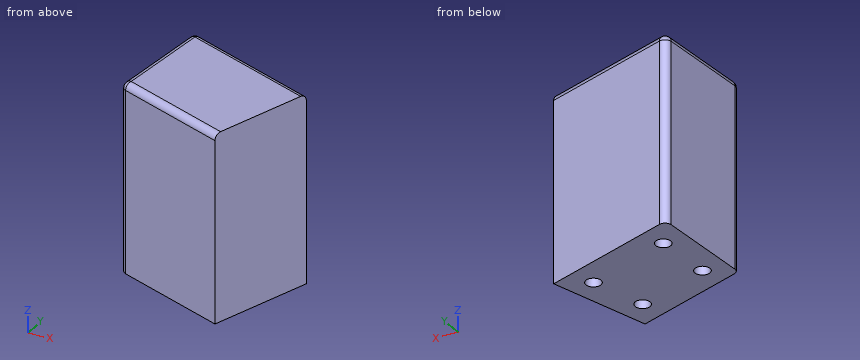
from build123d import *

# Parameters (mm, degrees)
BOSS_EXTRUDE1_DEPTH       = 74.025
FILLET1_R                 = 2.54
HOLE1_AT_2_COUNT          = 2
HOLE1_AT_2_PITCH          = 35.650433853
HOLE1_AT_3_COUNT          = 2
HOLE1_AT_3_PITCH          = 37.7542539
HOLE1_AT_4_COUNT          = 2
HOLE1_AT_4_PITCH          = 22.225
F_8_CLEARANCE_HOLE1_D     = 4.9149
F_8_CLEARANCE_HOLE1_DEPTH = 12.7
F_8_CLEARANCE_HOLE1_TIP   = 1.476584928


with BuildPart() as part:
    # Sketch1 → Boss-Extrude1 (new body)
    with BuildSketch(Plane.XY):
        Polygon((277.604402796, 374.816405204), (281.415155825, 417.005352091), (335.71810759, 399.192100573), (322.852981494, 359.973302076), align=None)
    extrude(amount=BOSS_EXTRUDE1_DEPTH)

    # Fillet1
    fillet1_edges = [part.edges().sort_by_distance(p)[0] for p in [
        (281.415155825, 417.005352091, 37.0125),
        (279.509779311, 395.910878647, 74.025),
        (300.228692145, 367.39485364, 74.025),
        (308.566631708, 408.098726332, 74.025),
        (277.604402796, 374.816405204, 37.0125),
    ]]
    fillet(fillet1_edges, radius=FILLET1_R)

    # Sketch3 → Hole1 (revolve, cut)
    with BuildSketch(Plane(origin=(323.698740376, 393.110483865, 0), x_dir=(0, 1, 0), z_dir=(1, 0, 0))):
        Polygon((0, 0), (0, 4.699), (2.8702, 4.699), (2.9972, 0), align=None)
    hole1 = revolve(axis=Axis((323.698740376, 393.110483865, 110), (0, 0, -1)), mode=Mode.SUBTRACT)

    # Hole1 at 2: Hole1 ×2
    with Locations(*[Vector(-0.950182883, 0.31169294, 0) * (i * HOLE1_AT_2_PITCH) for i in range(1, HOLE1_AT_2_COUNT)]):
        add(hole1, mode=Mode.SUBTRACT)

    # Hole1 at 3: Hole1 ×2
    with Locations(*[Vector(-0.951584848, -0.307386202, 0) * (i * HOLE1_AT_3_PITCH) for i in range(1, HOLE1_AT_3_COUNT)]):
        add(hole1, mode=Mode.SUBTRACT)

    # Hole1 at 4: Hole1 ×2
    with Locations(*[Vector(-0.31169294, -0.950182883, 0) * (i * HOLE1_AT_4_PITCH) for i in range(1, HOLE1_AT_4_COUNT)]):
        add(hole1, mode=Mode.SUBTRACT)

    # #8 Clearance Hole1
    with Locations(Plane(origin=(0, 0, 0), x_dir=(-1, 0, 0), z_dir=(0, 0, -1))):
        with Locations((-323.698740376, 393.110483865), (-289.824308357, 404.222472403), (-287.772364418, 381.505347156), (-316.771364786, 371.99266929)):
            Hole(F_8_CLEARANCE_HOLE1_D / 2, depth=F_8_CLEARANCE_HOLE1_DEPTH)
            with Locations((0, 0, -(F_8_CLEARANCE_HOLE1_DEPTH + F_8_CLEARANCE_HOLE1_TIP / 2))):  # 118° drill point
                Cone(0, F_8_CLEARANCE_HOLE1_D / 2, F_8_CLEARANCE_HOLE1_TIP, mode=Mode.SUBTRACT)


solid = part.part
Model file for the job. Use its own axes, mm. Round coordinates to 2 decimals unless told otherwise and drop trailing zeros. Order: outer loops, then holes, each group sorted by start corner. A loop starts at its lowest first (then second) coordinate and runs counter-clockwise, first axis right, second up.
(1) Band-saw the part on A-A (z = 69). List the corners of the cut face in (x, y).
(2) Drill centre lines: line 1 (Y direction, x = 316.5, z = 5); line 2 (X direction, y = 391.5, z = 7); line 3 (Z direction, x = 289, y = 384) (3 decimals). Where is each one in solid material? Low to high.
(3) Pin check, flat tips, straight feed: pin 1 (1.7 mm diameter, centred on x = 290, y = 404, fed in from -Z); pin 2 (3 mm diameter, centred on x = 289.82, y = 404.22, fed in from -Z); pin 3 (2 mm diameter, centred on y = 391, z = 53, fed in from +X). Stop position of each tip, or through.
Verdict:
1. outline: (277.79, 376.83) arc R2.54 ccw to (279.52, 374.19) - (322.85, 359.97) - (335.72, 399.19) - (284.45, 416.01) arc R2.54 ccw to (281.13, 413.83) - close
2. line 1: y = 362.06 to 369.55, 374.44 to 405.5
2. line 2: x = 279.11 to 321.84, 325.55 to 333.19
2. line 3: z = 4.699 to 74.025
3. pin 1: stops at z = 13.5
3. pin 2: stops at z = 13.27
3. pin 3: stops at x = 333.36
